Input: part model. Units: mm. Frame: model coordinates. A direction names the side the tool comes from. Round coordinates to 2 decimals unless told otherwise and drop trailing zeros. Loops run counter-clockwise (first coordinate to the right, second up) from the corner with the lowest first, then second, coordinate; pieces in that order, holes last.
1) Draft query along Z for faces 1 (the face through (35, 2, -32)), 2 (the face through (37, 3, 35)), 3 (the face through (-40, 3, 13)). Return one class per face: pulls with the +Z half, pulls with the -Z half, needs draft (parallel to the pull), parting line crosses it, or undercut.
2) Ray query, line 1 along X through (y, z) = (3.65, 2.5); line 2 along X through (y, z) = (0.2, -3). Return the intervals inside material, ascending.
3) Section A-A, the plane z = 2.5. Return loops of the section in (x, y), and give its area (3 significant figures).
4) Section B-B, the plane x = -37.5. State how many separate pieces and enclosed holes the cut face has, and give its area (3 significant figures).
5) First-contact query: pin 1 (2.5 mm diameter, centred on x = 36.5, y = 1.5, fed in from +Z); pin 2 (2.5 mm diameter, centred on y = 2, z = -13.5, fed in from +X). Flat tips, straight axial feed; report the tip coordinate or a pass-through.
6) Section D-D, the plane z = -33.5. Return loops of the section in (x, y), and give its area (3 significant figures).
7) Access query for faces 4 (the face through (-35, 2, -2)), 5 (the face through (-1, 5, -1)), 6 (the face through (37, 3, 25)), 7 (the face through (35, 2, 38)). Directions: +Z, -Z, +X, -X, +Y, -Y. A direction counts if a zero-diameter tool reaches every point of the face in a straight line with its end or side. Return the directions, or none.
from build123d import *

# Parameters (mm, degrees)
ESQUISSE1_W                     = 70
ESQUISSE1_H                     = 80
BOSS_EXTRU_1_DEPTH              = 5
ESQUISSE2_W                     = 5
ESQUISSE2_H                     = 5
BOSS_EXTRU_2_DEPTH              = 5
R_P_TITION_LIN_AIRE1_COUNT      = 2
R_P_TITION_LIN_AIRE1_PITCH      = 75
R_P_TITION_LIN_AIRE1_COUNT_DIR2 = 8
R_P_TITION_LIN_AIRE1_PITCH_DIR2 = 10
ESQUISSE3_R                     = 1.5
ENL_V_MAT_EXTRU_1_DEPTH         = 10


with BuildPart() as part:
    # Esquisse1 → Boss.-Extru.1 (new body)
    with BuildSketch(Plane(origin=(0, 0, 0), x_dir=(1, 0, 0), z_dir=(0, 1, 0))):
        Rectangle(ESQUISSE1_W, ESQUISSE1_H)
    extrude(amount=BOSS_EXTRU_1_DEPTH)

    # Esquisse2 → Boss.-Extru.2 (add)
    with BuildSketch(Plane(origin=(0, 5, 0), x_dir=(1, 0, 0), z_dir=(0, 1, 0))):
        with Locations((-37.5, 37.5)):
            Rectangle(ESQUISSE2_W, ESQUISSE2_H)
    boss_extru_2 = extrude(amount=-BOSS_EXTRU_2_DEPTH)

    # Répétition linéaire1: Boss.-Extru.2 2 × 8
    with Locations(*[(i * R_P_TITION_LIN_AIRE1_PITCH, 0, j * R_P_TITION_LIN_AIRE1_PITCH_DIR2) for i in range(R_P_TITION_LIN_AIRE1_COUNT) for j in range(R_P_TITION_LIN_AIRE1_COUNT_DIR2) if (i, j) != (0, 0)]):
        add(boss_extru_2)

    # Esquisse3 → Enlèv. mat.-Extru.1 (cut)
    with BuildSketch(Plane(origin=(0, 5, 0), x_dir=(1, 0, 0), z_dir=(0, 1, 0))):
        with Locations((-37.5, -2.5)):
            Circle(ESQUISSE3_R)
    enl_v_mat_extru_1 = extrude(amount=-ENL_V_MAT_EXTRU_1_DEPTH, mode=Mode.SUBTRACT)

    # Symétrie1: Enlèv. mat.-Extru.1 across plane
    add(enl_v_mat_extru_1.mirror(Plane(origin=(0, 0, 0), x_dir=(0, 0, 1), z_dir=(1, 0, 0))), mode=Mode.SUBTRACT)


solid = part.part
Final values:
1. face 1: undercut
1. face 2: pulls with the +Z half
1. face 3: needs draft
2. line 1: x = -40 to -39, -36 to 36, 39 to 40
2. line 2: x = -35 to 35
3. outline: (-40, 0) - (-39, 0) - (-39, 5) - (-40, 5) - close; (-36, 0) - (36, 0) - (36, 5) - (-36, 5) - close; (39, 0) - (40, 0) - (40, 5) - (39, 5) - close
3. area: 370 mm2
4. separate pieces: 9
4. enclosed holes: 0
4. area: 185 mm2
5. pin 1: stops at z = 35
5. pin 2: stops at x = 35
6. outline: (-35, 0) - (35, 0) - (35, 5) - (-35, 5) - close
6. area: 350 mm2
7. face 4: -X, +Y, -Y
7. face 5: +Z, -Z, +X, -X, +Y
7. face 6: +X, +Y, -Y
7. face 7: +Z, +X, +Y, -Y
